Autodesk Inventor part; units mm, degrees
ref_plane "YZ Plane" through (0, 0, 0) normal (1, 0, 0) x (0, 1, 0)
ref_plane "XZ Plane" through (0, 0, 0) normal (0, 1, 0) x (-1, 0, 0)
ref_plane "XY Plane" through (0, 0, 0) normal (0, 0, 1) x (1, 0, 0)
sketch "Эскиз1" plane through (0, 0, 0) normal (0, 0, 1) x (1, 0, 0)
  circle A0 centre (0, 0) radius 7
  dimension "d0" = 14
extrude "Выдавливание1" add sketch "Эскиз1" along normal blind 900
sketch "Эскиз2" plane through (0, 0, 0) normal (1, 0, 0) x (0, 1, 0)
  line L0 (7, 900) -> (-7, 900)
  line L1 (7, 0) -> (-7, 0)
  line L2 (0, 0) -> (0, 45)
  line L3 (0, 45) -> (7, 45)
  line L4 (7, 0) -> (7, 900)
  line L5 (7, 45) -> (7, 46)
  line L6 (7, 46) -> (0, 46)
  line L7 (0, 46) -> (0, 45)
  line L8 (0, 900) -> (0, 855)
  line L9 (0, 855) -> (7, 855)
  line L10 (7, 855) -> (7, 854)
  line L11 (0, -180) -> (0, 1080)
  line L12 (7, 854) -> (0, 854)
  line L13 (0, 855) -> (0, 854)
  line L14 (0, 46) -> (0, 45)
  line L15 (7, 46) -> (6, 46)
  line L16 (6, 46) -> (6, 45)
  line L17 (7, 855) -> (6, 855)
  line L18 (6, 854) -> (6, 855)
  dimension "d3" = 45
  dimension "d4" = 45
  dimension "d5" = 1
revolve "Вращение1" cut sketch "Эскиз2" angle 360 about axis through (0, 0, -10) along (0, 0, 1) contours L4 L12 L18 L9 | L4 L3 L16 L6
thread "Резьба1"
thread "Резьба2"
properties part number "Стяжка" material "Сталь, высокопрочная, низколегированная"
Geometry check sheet. Reference: the model listing, model coordinates, mm. A direction names the side the tool comes from. Give positions to 0.01 mm unless a question says otherwise; leave off trailing zeros. Loops run counter-clockwise (first coordinate to the right, second up) from the corner with the lowest first, then second, coordinate; pieces in that order, holes last. Notation, with made-up numbers: M -23,-24.75 L -6,-24.75 A13 ccw -6,-8.75 Z; hole C 27,66.5 d9. An arc over 180 degrees is marked long. Answer as a JSON object with one key per item and string values. Group by question number.
Item 1: Access from +Z, -Z, +X, -X, +Y, -Y to the whole of each face (thin tool, end or side, straight path). Record for faces 4 (the flat face through (-2, 6, 854)), 5 (the cylindrical face through (6.466, 2.681, 22.185)).
Item 2: Material ranges on L1, parallel to Z at x = -4.5, y = -5.25; L2, parallel to X at y = 3.5, z = 743; L3, parallel to X at y = 0.25, z = 44, recorded low to high.
Item 3: Sectioned sample at A-A on z = 148. Record the boundary of the cut face in (x, y).
Item 4: Mould release check, pull along Z, two halves, no side actions. Record for faces 1 (the flat face through (-2, 6, 45)), 2 (the cylindrical face through (6.466, 2.681, 877.185)), 3 (the flat face through (0, 0, 900)): pulls with the +Z half, pulls with the -Z half, needs draft (parallel to the pull), parting line crosses it, or undercut.
Item 5: Gauge pin test, flat ends, axial feed: pin 1 (3 mm diameter, centred on y = 3.5, z = 502, fed in from +X); pin 2 (1 mm diameter, centred on y = -5, z = 514, fed in from +X); pin 3 (2 mm diameter, centred on x = -5.5, z = 721.5, fed in from -Y). Record the tip position at first contact, or that the pin passes through.
Item 6: Sectioned sample at B-B on x = 3. Record the boundary of the cut face in (y, z).
Findings below:
{
 "1": {"face 4": "none", "face 5": "+Z, -Z"},
 "2": {"L1": "0 to 45, 46 to 854, 855 to 900", "L2": "-6.06 to 6.06", "L3": "-7 to 7"},
 "3": {"outline": "C 0,0 d14"},
 "4": {"face 1": "undercut", "face 2": "needs draft", "face 3": "pulls with the +Z half"},
 "5": {"pin 1": "x = 6.71", "pin 2": "x = 5.36", "pin 3": "y = -5.36"},
 "6": {"outline": "M -6.32,0 L 6.32,0 L 6.32,45 L 5.2,45 L 5.2,46 L 6.32,46 L 6.32,854 L 5.2,854 L 5.2,855 L 6.32,855 L 6.32,900 L -6.32,900 L -6.32,855 L -5.2,855 L -5.2,854 L -6.32,854 L -6.32,46 L -5.2,46 L -5.2,45 L -6.32,45 Z"}
}
